Source: CAD feature listing. Evaluate the final solid. Frame: model axes, mm. A direction names the side the tool comes from. Coordinates: 2 decimals unless noted, no trailing zeros. Order: outer loops, then holes, each group sorted by start corner. A loop starts at its lowest first (then second) coordinate and runs counter-clockwise, first axis right, second up.
```python
from build123d import *

# Parameters (mm, degrees)
SKETCH1_R           = 1.5
BOSS_EXTRUDE1_DEPTH = 10
SKETCH1_3_R         = 1.5
BOSS_EXTRUDE2_DEPTH = 33
BOSS_EXTRUDE3_DEPTH = 19


with BuildPart() as part:
    # Sketch1 → Boss-Extrude1 (new body)
    with BuildSketch(Plane(origin=(0, 0, 0), x_dir=(0, 0, -1), z_dir=(1, 0, 0))):
        Circle(SKETCH1_R)
    extrude(amount=-BOSS_EXTRUDE1_DEPTH)

    # Sketch1_3 → Boss-Extrude2 (add)
    with BuildSketch(Plane(origin=(0, 0, 0), x_dir=(0, 0, -1), z_dir=(1, 0, 0))):
        with BuildLine():
            ThreePointArc((4, 0), (3.645751311, 1.645751311), (2.645751311, 3))
            Line((2.645751311, 3), (-2.645751311, 3))
            ThreePointArc((-2.645751311, 3), (-1.645751311, -3.645751311), (4, 0))
        make_face()
        Circle(SKETCH1_3_R, mode=Mode.SUBTRACT)
        Circle(SKETCH1_3_R)
    extrude(amount=BOSS_EXTRUDE2_DEPTH)

    # Sketch1_4 → Boss-Extrude3 (add)
    with BuildSketch(Plane(origin=(0, 0, 0), x_dir=(0, 0, -1), z_dir=(1, 0, 0))):
        with BuildLine():
            Line((-2.645751311, 3), (2.645751311, 3))
            ThreePointArc((2.645751311, 3), (0, 4), (-2.645751311, 3))
        make_face()
    extrude(amount=BOSS_EXTRUDE3_DEPTH)


solid = part.part
```
1. Section query D-D on x = 0.5. Return loops of the section in (y, z), plus the area to 3 significant figures.
Findings:
outline: circle Ø8 at (0, 0)
area: 50.3 mm2
2. Access query for faces 1 (the face through (19, 3.4, 0)), 2 (the face through (33, 0, 0)), 3 (the face through (-4.93, 0.07, 1.5)). Directions: +Z, -Z, +X, -X, +Y, -Y. A direction counts if a zero-diameter tool reaches every point of the face in a straight line with its end or side. Return the directions, or none.
Findings:
face 1: +Z, -Z, +X, +Y
face 2: +Z, -Z, +X, +Y, -Y
face 3: -X
3. Section query A-A on z = 0. Return loops of the section in (x, y), plus the area to 3 significant figures.
Findings:
outline: (-10, -1.5) - (0, -1.5) - (0, -4) - (33, -4) - (33, 3) - (19, 3) - (19, 4) - (0, 4) - (0, 1.5) - (-10, 1.5) - close
area: 280 mm2
4. Pin query (flat end, axial travel): P1, Ø4, axis at x = 8, z = -3, coming from the +Y side; P2, Ø2.5, axis at x = 24.5, z = 0, coming from the +Y side. Return the tip coordinate at first contact, or that it passes through.
Findings:
P1: stops at y = 3.87
P2: stops at y = 3
5. Ray query, line 1 (X direction, y = 3.25, z = -0.5); line 2 (X direction, y = -1.5, z = -2.25); line 3 (Y direction, x = 10, z = -3). Return the intervals inside material, ascending.
Findings:
line 1: x = 0 to 19
line 2: x = 0 to 33
line 3: y = -2.65 to 2.65
6. Section query B-B on x = 30.5. Return loops of the section in (y, z).
Findings:
outline: (3, -2.65) - (3, 2.65) arc R4 ccw (long way) to start
7. Section query C-C on y = 2.5. Return loops of the section in (x, z).
Findings:
outline: (0, -3.12) - (33, -3.12) - (33, 3.12) - (0, 3.12) - close
